Autodesk Inventor part; units mm, degrees
ref_plane "YZ Plane" through (0, 0, 0) normal (1, 0, 0) x (0, 1, 0)
ref_plane "XZ Plane" through (0, 0, 0) normal (0, 1, 0) x (-1, 0, 0)
ref_plane "XY Plane" through (0, 0, 0) normal (0, 0, 1) x (1, 0, 0)
sketch "Sketch2" plane through (0, 0, 0) normal (0, 0, 1) x (1, 0, 0)
  circle A0 centre (0, 0) radius 3.175
  circle A1 centre (0, 0) radius 7.9375
  line L0 (-24.9815, -53.975) -> (30.0677, -53.975)
  line L1 (-24.9815, -53.975) -> (-36.2864, -11.7845)
  line L2 (-36.2864, -11.7845) -> (-3.9688, 6.8741)
  line L3 (20.5427, -47.625) -> (-13.5349, -47.625)
  line L4 (-13.5349, -47.625) -> (-22.3476, -14.7355)
  line L5 (-22.3476, -14.7355) -> (-5.9414, -5.2634)
  line L6 (-18.5621, -41.1307) -> (-23.4926, -22.7298) construction
  line L7 (-23.4926, -22.7298) -> (-29.6262, -24.3733) construction
  line L8 (-29.6262, -24.3733) -> (-24.6957, -42.7742) construction
  line L9 (-24.6957, -42.7742) -> (-18.5621, -41.1307) construction
  line L10 (-18.5621, -41.1307) -> (-29.6262, -24.3733) construction
  line L11 (-23.4926, -22.7298) -> (-24.6957, -42.7742) construction
  circle A2 centre (-29.6262, -24.3733) radius 1.7526
  circle A3 centre (-24.6957, -42.7742) radius 1.7526
  circle A4 centre (-21.0273, -31.9303) radius 1.7526
  line L12 (25.3052, -45.5804) -> (25.3052, -53.975) construction
  circle A5 centre (25.3052, -39.2375) radius 1.7526
  line L13 (0, 0) -> (-58.6646, -15.7191) construction
  line L14 (-24.0941, -32.752) -> (-30.6681, -8.2175) construction
  circle A6 centre (25.3052, -39.2375) radius 4.7625
  line L15 (30.0677, -39.2375) -> (30.0677, -53.975)
  line L16 (20.5427, -39.2375) -> (20.5427, -47.625)
  line L17 (-30.2278, -34.3955) -> (-17.9605, -31.1085) construction
  line L18 (-24.9815, -53.975) -> (-113.8815, -53.975)
  circle A7 centre (-9.9632, -48.6877) radius 1.7526
  line L19 (-9.9632, -48.6877) -> (-25.2973, -52.7964) construction
  line L20 (25.3052, -39.2375) -> (24.0725, -34.6373) construction
  line L21 (-31.2313, -30.6503) -> (-77.8688, -47.625)
  line L22 (-77.8688, -47.625) -> (-26.6829, -47.625)
  line L23 (-9.9632, -48.6877) -> (-10.4168, -46.9948) construction
  circle A8 centre (25.3052, -39.2375) radius 1.7526
  circle A9 centre (25.3052, -39.2375) radius 4.7625
  line L24 (17.994, -39.5531) -> (8.9547, -5.8181)
  line L25 (8.9547, -5.8181) -> (-22.4801, -14.241) construction
  line L26 (-22.4801, -14.241) -> (-13.4409, -47.976) construction
  line L27 (-0.2817, -44.45) -> (17.994, -39.5531)
  line L28 (17.994, -39.5531) -> (-22.4801, -14.241) construction
  line L29 (8.9547, -5.8181) -> (-13.4409, -47.976) construction
  line L30 (6.9477, 3.8384) -> (29.4738, -36.9345)
  line L31 (2.0544, -7.667) -> (8.9547, -5.8181)
  circle A10 centre (-9.9632, -48.6877) radius 4.7625 construction
  line L32 (-0.2817, -44.45) -> (-14.3857, -44.45)
  line L33 (-113.8815, -53.975) -> (-32.8811, -24.4933)
  circle A11 centre (-54.7623, -40.9695) radius 1.7526
  circle A12 centre (-54.7623, -40.9695) radius 7.9375
  line L34 (-54.7623, -40.9695) -> (-56.8404, -33.2138) construction
  line L35 (-25.8322, -50.8) -> (-105.1582, -50.8) construction
  circle A13 centre (-47.625, -50.8) radius 1.7526
  circle A14 centre (-57.15, -50.8) radius 1.7526
  circle A15 centre (-66.675, -50.8) radius 1.7526
  circle A16 centre (-76.2, -50.8) radius 1.7526
  circle A17 centre (12.7, -50.8) radius 1.7526
  line L36 (0.6918, 7.9073) -> (27.1694, 5.5908)
  circle A18 centre (26.8927, 2.4279) radius 1.7526
  circle A19 centre (26.8927, 2.4279) radius 3.175
  line L37 (8.6038, 0.8408) -> (26.616, -0.735)
  circle A20 centre (17.4039, 3.258) radius 1.7526
  line L38 (-9.9632, -48.6877) -> (-9.9632, -48.6877) construction
  point P0 (7.667, 2.0544)
  point P1 (0.4795, -7.923)
  point P2 (-24.0941, -32.752)
  point P3 (-2.2431, -26.897)
  point P4 (-2.2431, -26.897)
  point P5 (-12.1309, -47.625)
  point P6 (-15.5208, -47.3441)
  point P7 (29.4738, -36.9345)
  point P8 (-14.3857, -44.45)
  point P9 (-9.6568, -46.9621)
  point P10 (-9.6568, -46.9621)
  point P11 (-48.0301, -36.7646)
  point P12 (-59.0876, -47.625)
  point P13 (-62.6223, -42.0757)
  point P14 (-50.4369, -47.625)
  point P15 (13.8439, -8.6439)
  point P16 (24.4605, 0.387)
  point P17 (23.7298, 2.7046)
  dimension "d7" = 15.875
  dimension "d40" = 3.5052
  dimension "d6" = 6.35
  dimension "Angle_Mount" = 105
  dimension "d17" = 105
  dimension "d19" = 9.525
  dimension "d20" = 12.7
  dimension "d24" = 19.05
  dimension "d25" = 6.35
  dimension "d26" = 3.5052
  dimension "d27" = 3.5052
  dimension "d28" = 3.5052
  dimension "d29" = 6.35
  dimension "d33" = 3.5052
  dimension "d35" = 31.75
  dimension "d37" = 9.525
  dimension "d38" = 25.4
  dimension "d39" = 53.975
  dimension "d41" = 44.45
  dimension "Rail_Offset" = 36.5125
  dimension "d45" = 6.35
  dimension "d48" = 22.225
  dimension "d49" = 3.5052
  dimension "d51" = 9.525
  dimension "d52" = 32.5438
  dimension "d53" = 34.925
  dimension "d54" = 9.525
  dimension "d56" = 9.525
  dimension "d58" = 6.35
  dimension "d60" = 20
  dimension "d61" = 88.9
  dimension "d69" = 31.75
  dimension "d71" = 3.5052
  dimension "d72" = 15.875
  dimension "d74" = 3.175
  dimension "d75" = 3.5052
  dimension "d76" = 47.625
  dimension "d79" = 9.525
  dimension "d84" = 3.5052
  dimension "d85" = 60.325
  dimension "d86" = 145
  dimension "d87" = 3.5052
  dimension "d88" = 6.35
  dimension "d101" = 9.525
extrude "Extrusion2" add sketch "Sketch2" along normal blind 6.35 contours A1 | A1 L30 A6 L16 L3 A7 L4 L32 L27 L24 L31 | L5 L4 L3 A7 L16 A6 L15 L0 L1 L2 A1 | A6 | L1 L21 A12 L22 L18 L33 | A7 L3 | L3 A7 | A12 L22 L21 A11 | L21 A11 A12 | A12 L22 | A12 L22 L21
fillet "Fillet1" radius 3.175 15 edges at (-22.3476, -14.7355, 3.175) (-5.9414, -5.2634, 3.175) (8.9547, -5.8181, 3.175) (17.994, -39.5531, 3.175) (-14.3857, -44.45, 3.175) (-0.2817, -44.45, 3.175) (30.0677, -53.975, 3.175) (-36.2864, -11.7845, 3.175) (-26.6829, -47.625, 3.175) (-50.4369, -47.625, 3.175) (-48.0301, -36.7646, 3.175) (-31.2313, -30.6503, 3.175) (-32.8811, -24.4933, 3.175) (-113.8815, -53.975, 3.175) (6.9477, 3.8384, 3.175)
properties part number "Uprights" material "Aluminum 6061"
Read the model definition and answer for the solid it produces. Units are mm, in the model's axes. A direction names the side the tool comes from. Coordinates: 2 decimals unless noted, no trailing zeros. Loops run counter-clockwise (first coordinate to the right, second up) from the corner with the lowest first, then second, coordinate; pieces in that order, holes last.
Q1. Which of the six approach directions +Z, -Z, +X, -X, +Y, -Y give full straight-line access (tool end or side, diameter ignored) to faces 4 (the face through (13.526, -22.879, 3.131)), 5 (the face through (-35, -53.975, 3))?
Q2. The part is cut by section A-A on x = 12.7. Write down the section's boundary in (y, z) (3 decimals).
Q3. The part is cut by section D-D on z = 1. Give the number of separate pieces and of enclosed holes in the cut face, and give its area (3 significant figures).
Q4. The mould has two halves that part along X. Classify faces 1 (the face through (-68.066, -49.734, 3.131)), 2 (the face through (18.05, -16.26, 3.13)), 3 (the face through (-19.284, -1.968, 3.131)): +X half, -X half, draft (parallel to the pull), parting line (faces both ways), or undercut.
Q5. Consider probe 1 along X at (y, z) = (-25, 1.25); probe 2 along Y at (x, z) = (-46.5, 4.5) (3 decimals); probe 3 along X at (y, z) = (-50, 3.75). Determine where each line is inside the solid, lowest interval first.
Q6. Each of these flat-tipped pins is pushed along its axis until it touches: pin 1 Ø3 at (x, y) = (-57.15, -50.8) entering from +Z; pin 2 Ø1.9 at (x, z) = (-4.5, 2.5) entering from +Y; pin 3 Ø1.9 at (x, z) = (-39, 2) entering from +Y; pin 4 Ø2 at (x, z) = (-69, 1.5) entering from +Y. Where does it stop, or does it pass through?
Q7. The part is cut by section C-C on x = -76.2. Write down the section's boundary in (y, z) (3 decimals), and give its area (3 significant figures).
Q8. The part is cut by section B-B on y = 0. Write down the section's boundary in (x, z) (3 decimals), and give its area (3 significant figures).
Results below:
1. face 4: +Z, -Z
1. face 5: +Z, -Z, +X, -X, -Y
2. outline: (-53.975, 0) - (-52.553, 0) - (-52.553, 6.35) - (-53.975, 6.35) - close; (-49.047, 0) - (-40.972, 0) - (-40.972, 6.35) - (-49.047, 6.35) - close; (-19.796, 0) - (-6.573, 0) - (-6.573, 6.35) - (-19.796, 6.35) - close
3. separate pieces: 1
3. enclosed holes: 13
3. area: 2,680 mm2
4. face 1: undercut
4. face 2: +X half
4. face 3: -X half
5. probe 1: x = -34.74 to -31.26, -27.99 to -19.6, 14.09 to 22.88
5. probe 2: y = -53.975 to -52.144, -49.456 to -46.648, -36.821 to -29.45
5. probe 3: x = -98.95 to -77.76, -74.64 to -68.23, -65.12 to -58.71, -55.59 to -49.18, -46.07 to 11.14, 14.26 to 30.07
6. pin 1: passes through
6. pin 2: stops at y = 7.1
6. pin 3: stops at y = -26.37
6. pin 4: stops at y = -37.28
7. outline: (-53.975, 0) - (-52.553, 0) - (-52.553, 6.35) - (-53.975, 6.35) - close; (-49.047, 0) - (-40.26, 0) - (-40.26, 6.35) - (-49.047, 6.35) - close
7. area: 64.8 mm2
8. outline: (-15.875, 0) - (-3.175, 0) - (-3.175, 6.35) - (-15.875, 6.35) - close; (3.175, 0) - (9.068, 0) - (9.068, 6.35) - (3.175, 6.35) - close
8. area: 118 mm2
